from build123d import *

# Parameters (mm, degrees)
SKETCH1_R           = 15
BOSS_EXTRUDE1_DEPTH = 6


with BuildPart() as part:
    # Sketch1 → Boss-Extrude1 (new body)
    with BuildSketch(Plane.XY):
        Circle(SKETCH1_R)
        with BuildLine():
            Line((-1.285714286, 5.860626142), (-1.285714286, 11.930923635))
            ThreePointArc((-1.285714286, 11.930923635), (-8.485281374, 8.485281374), (-11.930923635, 1.285714286))
            Line((-11.930923635, 1.285714286), (-5.860626142, 1.285714286))
            ThreePointArc((-5.860626142, 1.285714286), (-4.242640687, 4.242640687), (-1.285714286, 5.860626142))
        make_face(mode=Mode.SUBTRACT)
        with BuildLine():
            Line((1.285714286, 5.860626142), (1.285714286, 11.930923635))
            ThreePointArc((1.285714286, 11.930923635), (8.485281374, 8.485281374), (11.930923635, 1.285714286))
            Line((11.930923635, 1.285714286), (5.860626142, 1.285714286))
            ThreePointArc((5.860626142, 1.285714286), (4.242640687, 4.242640687), (1.285714286, 5.860626142))
        make_face(mode=Mode.SUBTRACT)
        with BuildLine():
            Line((-1.285714286, -11.930923635), (-1.285714286, -5.860626142))
            ThreePointArc((-1.285714286, -5.860626142), (-4.164035651, -4.319815632), (-5.809475019, -1.5))
            Line((-5.809475019, -1.5), (-11.9058809, -1.5))
            ThreePointArc((-11.9058809, -1.5), (-8.408661478, -8.561215577), (-1.285714286, -11.930923635))
        make_face(mode=Mode.SUBTRACT)
        with BuildLine():
            Line((1.285714286, -11.930923635), (1.285714286, -5.860626142))
            ThreePointArc((1.285714286, -5.860626142), (4.164035651, -4.319815632), (5.809475019, -1.5))
            Line((5.809475019, -1.5), (11.9058809, -1.5))
            ThreePointArc((11.9058809, -1.5), (8.408661478, -8.561215577), (1.285714286, -11.930923635))
        make_face(mode=Mode.SUBTRACT)
        with BuildLine():
            Line((-1.984313483, -2.25), (1.984313483, -2.25))
            ThreePointArc((1.984313483, -2.25), (0, 3), (-1.984313483, -2.25))
        make_face(mode=Mode.SUBTRACT)
    extrude(amount=BOSS_EXTRUDE1_DEPTH)


solid = part.part
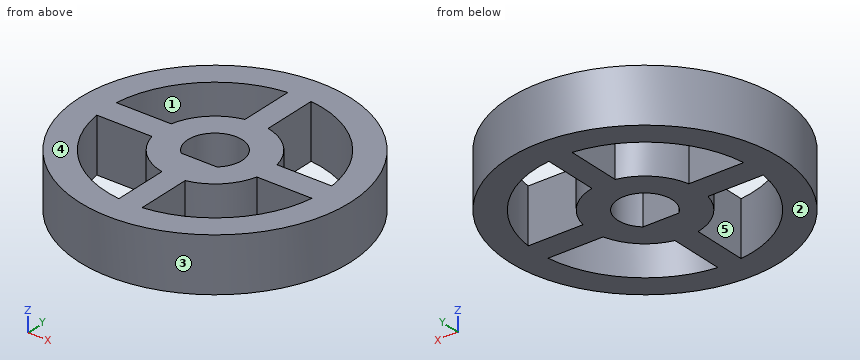
Verification items for the finished model (mm, model axes). Face numbers are marked on the shaded views. A direction names the side the tool comes from. Give positions to 0.01 mm unless a question says otherwise; leave off trailing zeros. Write each loop counter-clockwise with the first axis right and the second up, starting at its lowest first coordinate (ties: lowest second). Pieces come first, ordered by that corner, then holes. Notation, with made-up numbers: (76, 46.5) - (89, 46.5) arc R18 ccw to (89, 57.5) - close; hole circle Ø8 at (-29, -34). An arc over 180 degrees is marked (long way). Answer as CSV lines item,"result". Start each with the question number.
1. Depth check by flat-ended pin: pin 1 (2 mm diameter, centred on y = 2.5, z = 4.5, fed in from -X); pin 2 (1.8 mm diameter, centred on y = 9.5, z = 3.5, fed in from -X); pin 3 (1.8 mm diameter, centred on x = -10, z = 4, fed in from +Y). Enter the tip coordinate at first touch or a pass-through.
2. Sectioned sample at B-B (x = 0). Record the boundary of the cut face in (y, z), then the cut area to 4 significant figures.
3. Draft check along Y on the marked faces 1, 2 and 3. Enter one of: pulls with the +Y half, pulls with the -Y half, needs draft (parallel to the pull), parting line crosses it, or undercut.
4. Sectioned sample at A-A (y = 0). Record the boundary of the cut face in (x, z), then the cut area to 3 significant figures.
5. Sectioned sample at D-D (y = -4.25). Record the boundary of the cut face in (x, z).
6. Thickness scan on line 1 (Y direction, x = 10.25, z = 1.8); line 2 (Y direction, x = 5.25, z = 2.5); line 3 (X direction, y = 11, z = 5.1). Record the ranges inside material, lowest first.
7. Sectioned sample at C-C (z = 3.4). Record the boundary of the cut face in (x, y), then the cut area to 3 significant figures.
8. Set-up check for the marked faces 4 and 5: record each of +Z, -Z, +X, -X, +Y, -Y from which the full face is reachable in a straight line by a thin tool's end or side.
Derived:
1,pin 1,"x = -14.92"
1,pin 2,"x = -12.29"
1,pin 3,"y = 11.92"
2,outline,"(-15, 0) - (-2.25, 0) - (-2.25, 6) - (-15, 6) - close; (3, 0) - (15, 0) - (15, 6) - (3, 6) - close"
2,area,"148.5 mm²"
3,face 1,"undercut"
3,face 2,"needs draft"
3,face 3,"parting line crosses it"
4,outline,"(-15, 0) - (-3, 0) - (-3, 6) - (-15, 6) - close; (3, 0) - (15, 0) - (15, 6) - (3, 6) - close"
4,area,"144 mm²"
5,outline,"(-14.39, 0) - (-11.22, 0) - (-11.22, 6) - (-14.39, 6) - close; (-4.24, 0) - (4.24, 0) - (4.24, 6) - (-4.24, 6) - close; (11.22, 0) - (14.39, 0) - (14.39, 6) - (11.22, 6) - close"
6,line 1,"-10.95 to -6.24, -1.5 to 1.29, 6.24 to 10.95"
6,line 2,"-14.05 to -10.79, -2.9 to 2.9, 10.79 to 14.05"
6,line 3,"-10.2 to -4.8, -1.29 to 1.29, 4.8 to 10.2"
7,outline,"circle Ø30 at (0, 0); hole (-11.93, 1.29) - (-5.86, 1.29) arc R6 cw to (-1.29, 5.86) - (-1.29, 11.93) arc R12 ccw to start; hole (-11.91, -1.5) arc R12 ccw to (-1.29, -11.93) - (-1.29, -5.86) arc R6 cw to (-5.81, -1.5) - close; hole (-1.98, -2.25) - (1.98, -2.25) arc R3 ccw (long way) to start; hole (1.29, -11.93) arc R12 ccw to (11.91, -1.5) - (5.81, -1.5) arc R6 cw to (1.29, -5.86) - close; hole (1.29, 5.86) arc R6 cw to (5.86, 1.29) - (11.93, 1.29) arc R12 ccw to (1.29, 11.93) - close"
7,area,"406 mm²"
8,face 4,"+Z, +X, -X, +Y, -Y"
8,face 5,"+Z, -Z"
